Design review of the part shown in the three views and the two pictorial views. Dimensions are in mm from the part's minimum x, y and z. Coordinates: 2 decimals unless noted, no trailing zeros. Loops run counter-clockwise (first coordinate to the right, second up) from the corner with the lowest first, then second, coordinate; pieces in that order, holes last. Notation, with made-up numbers: M 60.5,82.25 L 79.5,82.25 A11 cw 79.5,97.25 Z; hole C 25.5,65.25 d11. An arc over 180 degrees is marked long. Use one line per item in the form item = value.
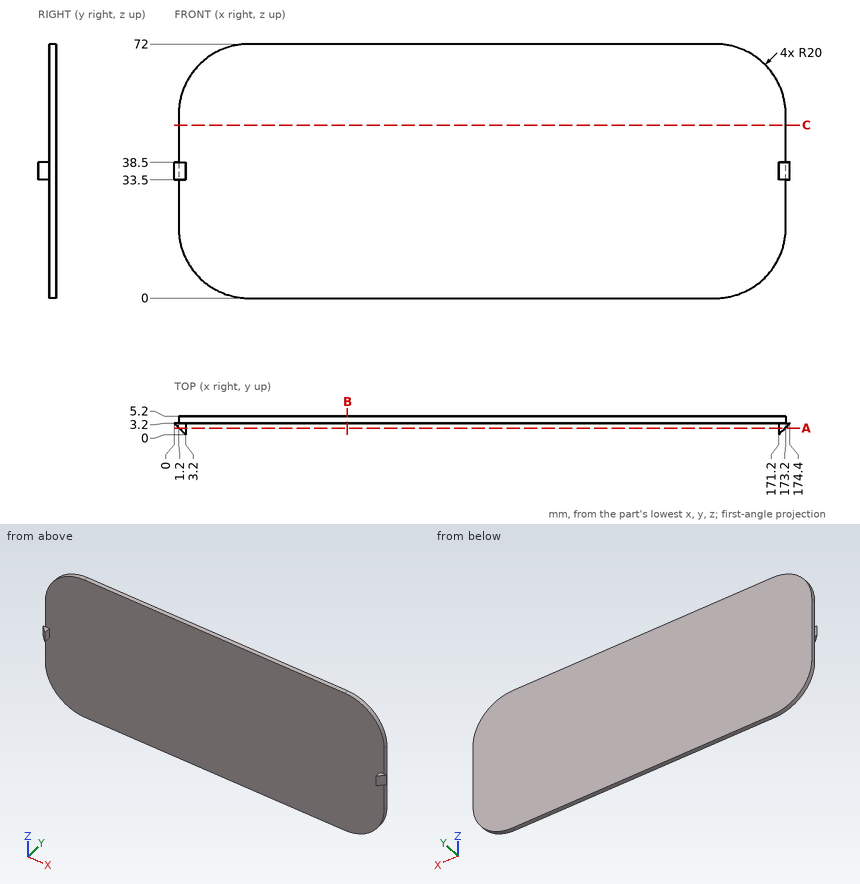
1. Add section A-A (y = 1.8). State the section outline as (x, z) points.
Response values:
outline = M 1.4,33.5 L 3.2,33.5 L 3.2,38.5 L 1.4,38.5 Z; M 171.2,33.5 L 173,33.5 L 173,38.5 L 171.2,38.5 Z
2. Add section B-B (x = 49). State the section outline as (y, z) points, then the cut area to 3 significant figures.
Response values:
outline = M 3.2,0 L 5.2,0 L 5.2,72 L 3.2,72 Z
area = 144 mm^2
3. Insertion check: P1, Ø2.5, axis at x = 1, y = 1, coming from the -Z side; P2, Ø2.5, axis at x = 172, y = 1, coming from the +Z side; P3, Ø2.5, axis at y = 1.5, z = 36, coming from the -X side. Each pin has a flat end and moves straight along its axis. Give the tip position at first contact, or say it passes through.
Response values:
P1 = 33.5
P2 = 38.5
P3 = 0.45
4. Add section C-C (z = 49). State the section outline as (x, y) points.
Response values:
outline = M 1.2,3.2 L 173.2,3.2 L 173.2,5.2 L 1.2,5.2 Z
5. Wall thickness on line 1 along X through (y, z) = (4.6, 19.5); line 2 along Y through (x, z) = (104, 30); line 3 along X through (y, z) = (4.25, 59.5): over which ranges is each line inside the solid? List them lowest first. Write a range as from..to.
Response values:
line_1 = 1.21..173.19
line_2 = 3.2..5.2
line_3 = 2.66..171.74
